For this review, take the finished solid that the model builds, in its own axes (mm). A direction names the side the tool comes from. Coordinates: 2 decimals unless noted, no trailing zeros. Write each loop counter-clockwise with the first axis right and the second up, starting at its lowest first coordinate (ties: lowest second). Pieces come first, ordered by that corner, then holes.
1) To check wall thickness, follow line 1 along X through (y, z) = (5.15, 18.5); line 2 along Z through (x, y) = (-9.75, 5.25); line 3 along Z through (x, y) = (-10, 3.05). State the ranges of each line that lie inside material, in increasing order.
2) Mouldability with a two-part tool opening along X and no side actions: class faces 5 (the face through (10, 0, 1)), 6 (the face through (0, 3, -12)) as pulls with the +X half, pulls with the -X half, needs draft (parallel to the pull), parting line crosses it, or undercut.
3) We need section D-D on y = 3.25. Give the number of separate pieces and of enclosed holes in the cut face, then the cut area to 3 significant figures.
4) We need section C-C on x = 10.75. Write out the cut boundary in (y, z), then the cut area to 3 significant figures.
5) We need section A-A on x = 0. Write out the cut boundary in (y, z).
6) For faces 1 (the face through (2.1, 6, 2)), 2 (the face through (12, 4.5, 18)), 3 (the face through (0, 2.1, -15.8)), 4 (the face through (0, 3, 16.9)), list the 3-axis set-ups (+Z, -Z, +X, -X, +Y, -Y) from which the entire face can be reached by the end or side of a thin tool; tool diameter is ignored.
7) We need section B-B on z = 11. Write out the cut boundary in (x, y).
8) Insertion check: P1, Ø1.5, axis at x = 3.5, z = -9.5, coming from the -Y side; P2, Ø2.5, axis at x = -10, z = 18.5, coming from the -Y side; P3, Ø2, axis at x = 10.5, z = 19, coming from the +Y side. Each pin has a flat end and moves straight along its axis. Give the tip position at first contact, or say it passes through.
from build123d import *

# Parameters (mm, degrees)
SKETCH1_W           = 30
SKETCH1_H           = 47
BOSS_EXTRUDE1_DEPTH = 6.5
BOSS_EXTRUDE2_DEPTH = 3
SKETCH3_R           = 2.1
CUT_EXTRUDE1_DEPTH  = 50
FILLET1_R           = 5
SKETCH4_R           = 4.1
CUT_EXTRUDE2_DEPTH  = 3.1
SKETCH5_W           = 10
SKETCH5_H           = 26
CUT_EXTRUDE3_DEPTH  = 5
SKETCH9_R           = 4.1
CUT_EXTRUDE4_DEPTH  = 3.1
SKETCH10_R          = 5
CUT_EXTRUDE5_DEPTH  = 6
SKETCH11_R          = 1.5
CUT_EXTRUDE6_DEPTH  = 7.5
SKETCH12_R          = 3.5
CUT_EXTRUDE7_DEPTH  = 2
CUT_EXTRUDE8_DEPTH  = 2.5


with BuildPart() as part:
    # Sketch1 → Boss-Extrude1 (new body)
    with BuildSketch(Plane(origin=(0, 0, 0), x_dir=(1, 0, 0), z_dir=(0, 1, 0))):
        Rectangle(SKETCH1_W, SKETCH1_H)
    extrude(amount=BOSS_EXTRUDE1_DEPTH)

    # Sketch2 → Boss-Extrude2 (add)
    with BuildSketch(Plane.XY.offset(23.5)):
        with BuildLine():
            Line((5, 0), (-5, 0))
            ThreePointArc((-5, 0), (0, 5), (5, 0))
        make_face()
    extrude(amount=BOSS_EXTRUDE2_DEPTH)

    # Sketch3 → Cut-Extrude1 (cut)
    with BuildSketch(Plane.XY.offset(26.5)):
        Circle(SKETCH3_R)
    extrude(amount=-CUT_EXTRUDE1_DEPTH, mode=Mode.SUBTRACT)

    # Fillet1
    fillet1_edges = [part.edges().sort_by_distance(p)[0] for p in [
        (15, 3.25, 23.5),
        (-15, 3.25, 23.5),
    ]]
    fillet(fillet1_edges, radius=FILLET1_R)

    # Sketch4 → Cut-Extrude2 (cut)
    with BuildSketch(Plane.XY.offset(20)):
        Circle(SKETCH4_R)
    extrude(amount=-CUT_EXTRUDE2_DEPTH, mode=Mode.SUBTRACT)

    # Sketch5 → Cut-Extrude3 (cut)
    with BuildSketch(Plane.XZ):
        with Locations((0, 2.5)):
            Rectangle(SKETCH5_W, SKETCH5_H)
    extrude(amount=-CUT_EXTRUDE3_DEPTH, mode=Mode.SUBTRACT)

    # Sketch9 → Cut-Extrude4 (cut)
    with BuildSketch(Plane.XY.offset(-12)):
        Circle(SKETCH9_R)
    extrude(amount=-CUT_EXTRUDE4_DEPTH, mode=Mode.SUBTRACT)

    # Sketch10 → Cut-Extrude5 (cut)
    with BuildSketch(Plane.XY.offset(-16.6)):
        Circle(SKETCH10_R)
    extrude(amount=-CUT_EXTRUDE5_DEPTH, mode=Mode.SUBTRACT)

    # Sketch11 → Cut-Extrude6 (cut, through all)
    with BuildSketch(Plane.XZ):
        with Locations((10, 18.5)):
            Circle(SKETCH11_R)
        with Locations((10, -19.5)):
            Circle(SKETCH11_R)
        with Locations((-10, -19.5)):
            Circle(SKETCH11_R)
        with Locations((-10, 18.5)):
            Circle(SKETCH11_R)
    extrude(amount=-CUT_EXTRUDE6_DEPTH, mode=Mode.SUBTRACT)

    # Sketch12 → Cut-Extrude7 (cut)
    with BuildSketch(Plane(origin=(0, 6.5, 0), x_dir=(1, 0, 0), z_dir=(0, 1, 0))):
        with Locations((-10, 19.5)):
            Circle(SKETCH12_R)
        with Locations((10, 19.5)):
            Circle(SKETCH12_R)
        with Locations((10, -18.5)):
            Circle(SKETCH12_R)
        with Locations((-10, -18.5)):
            Circle(SKETCH12_R)
    extrude(amount=-CUT_EXTRUDE7_DEPTH, mode=Mode.SUBTRACT)

    # Sketch13 → Cut-Extrude8 (cut, through all)
    with BuildSketch(Plane.XZ.offset(-5)):
        Polygon((0, -10.5), (2.1, -10.5), (2.1, 15.5), (-2.1, 15.5), (-2.1, -10.5), align=None)
    extrude(amount=-CUT_EXTRUDE8_DEPTH, mode=Mode.SUBTRACT)


solid = part.part
Result:
1. line 1: x = -15 to -13.5, -6.5 to 6.5, 13.5 to 15
1. line 2: z = -23.5 to -22.99, -16.01 to 15.01, 21.99 to 23.5
1. line 3: z = -23.5 to -21, -18 to 17, 20 to 23.5
2. face 5: needs draft
2. face 6: undercut
3. separate pieces: 1
3. enclosed holes: 8
3. area: 1,060 mm2
4. outline: (0, -23.5) - (6.5, -23.5) - (6.5, -22.92) - (4.5, -22.92) - (4.5, -20.8) - (0, -20.8) - close; (0, -18.2) - (4.5, -18.2) - (4.5, -16.08) - (6.5, -16.08) - (6.5, 15.08) - (4.5, 15.08) - (4.5, 17.2) - (0, 17.2) - close; (0, 19.8) - (4.5, 19.8) - (4.5, 21.92) - (6.5, 21.92) - (6.5, 23.44) - (0, 23.44) - close
4. area: 254 mm2
5. outline: (2.1, -23.5) - (6.5, -23.5) - (6.5, -10.5) - (2.1, -10.5) - (2.1, -12) - (4.1, -12) - (4.1, -15.1) - (2.1, -15.1) - (2.1, -16.6) - (5, -16.6) - (5, -22.6) - (2.1, -22.6) - close; (2.1, 15.5) - (6.5, 15.5) - (6.5, 23.5) - (5, 23.5) - (5, 26.5) - (2.1, 26.5) - (2.1, 20) - (4.1, 20) - (4.1, 16.9) - (2.1, 16.9) - close
6. face 1: +Y, -Y
6. face 2: +Y
6. face 3: +Z, -Z, -Y
6. face 4: -Y
7. outline: (-15, 0) - (-5, 0) - (-5, 5) - (-2.1, 5) - (-2.1, 6.5) - (-15, 6.5) - close; (2.1, 5) - (5, 5) - (5, 0) - (15, 0) - (15, 6.5) - (2.1, 6.5) - close
8. P1: stops at y = 5
8. P2: passes through
8. P3: stops at y = 4.5
